Could you check a few things on this drawing? It's one solid part, dimensions in mm from its lowest x, y, z. Give positions to 0.01 mm unless a question says otherwise; leave off trailing zeros. Order: outer loops, then holes, each group sorted by start corner. A loop starts at its lowest first (then second) coordinate and runs counter-clockwise, first axis right, second up.
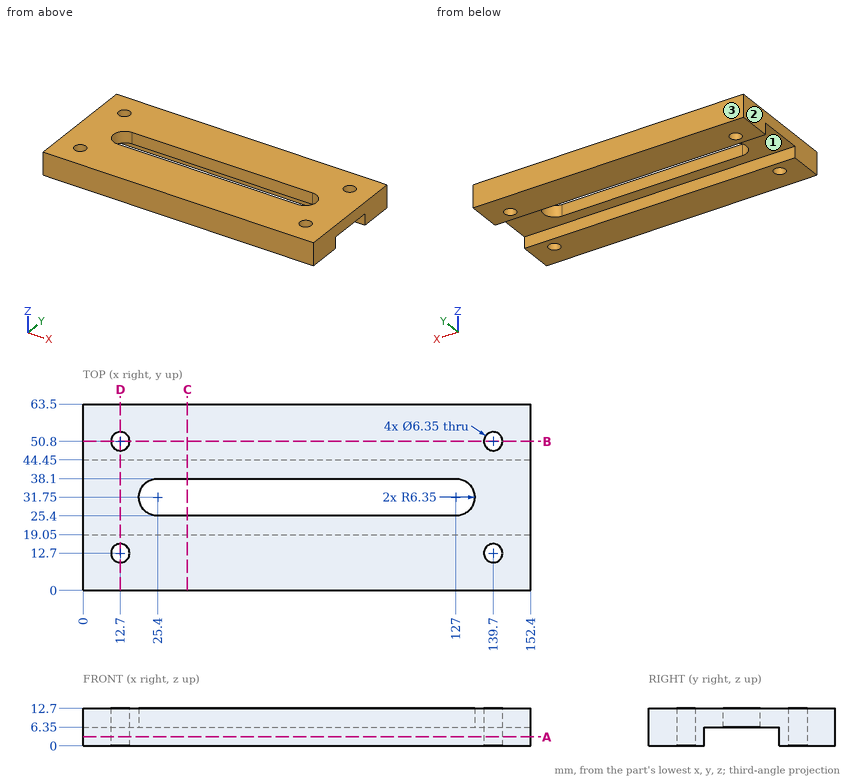
Q1. If we section it at C-C on x = 35.5: List the corners of the cut face in (y, z) for me.
Filled sheet:
outline: (0, 0) - (19.05, 0) - (19.05, 6.35) - (25.4, 6.35) - (25.4, 12.7) - (0, 12.7) - close; (38.1, 6.35) - (44.45, 6.35) - (44.45, 0) - (63.5, 0) - (63.5, 12.7) - (38.1, 12.7) - close
Q2. If we section it at D-D on x = 12.7: List the corners of the cut face in (y, z) for me (3 decimals), plus the area to 3 significant figures.
Filled sheet:
outline: (0, 0) - (9.525, 0) - (9.525, 12.7) - (0, 12.7) - close; (15.875, 0) - (19.05, 0) - (19.05, 6.35) - (44.45, 6.35) - (44.45, 0) - (47.625, 0) - (47.625, 12.7) - (15.875, 12.7) - close; (53.975, 0) - (63.5, 0) - (63.5, 12.7) - (53.975, 12.7) - close
area: 484 mm2
Q3. Thinking about a two-plate mould opening in Y: for the marked faces 1, 2 and 3, which applies, released by +Y, released by -Y, zero draft, split by the parting line, or undercut?
Filled sheet:
face 1: undercut
face 2: zero draft
face 3: released by +Y
Q4. I'm going to push a flat-ended pin straight in: P1, Ø5, axis at x = 12.7, y = 50.8, coming from the -Z side. Where does the tip first touch, or does it pass through?
Filled sheet:
P1: passes through
Q5. I need wall thicknesses on L1, parallel to Y at x = 139.7, z = 4.5 (3 decimals); L2, parallel to Y at x = 139.7, z = 8 (3 decimals); L3, parallel to Y at x = 112, z = 8.25. Which ranges of each line are inside material? Lowest first, please.
Filled sheet:
L1: y = 0 to 9.525, 15.875 to 19.05, 44.45 to 47.625, 53.975 to 63.5
L2: y = 0 to 9.525, 15.875 to 47.625, 53.975 to 63.5
L3: y = 0 to 25.4, 38.1 to 63.5
Q6. If we section it at A-A on z = 3: List the corners of the cut face in (x, y) for me (3 decimals).
Filled sheet:
outline: (0, 0) - (152.4, 0) - (152.4, 19.05) - (0, 19.05) - close; (0, 44.45) - (152.4, 44.45) - (152.4, 63.5) - (0, 63.5) - close; hole circle Ø6.35 at (12.7, 12.7); hole circle Ø6.35 at (12.7, 50.8); hole circle Ø6.35 at (139.7, 12.7); hole circle Ø6.35 at (139.7, 50.8)
Q7. If we section it at B-B on y = 50.8: List the corners of the cut face in (x, z) for me (3 decimals).
Filled sheet:
outline: (0, 0) - (9.525, 0) - (9.525, 12.7) - (0, 12.7) - close; (15.875, 0) - (136.525, 0) - (136.525, 12.7) - (15.875, 12.7) - close; (142.875, 0) - (152.4, 0) - (152.4, 12.7) - (142.875, 12.7) - close
